```python
from build123d import *

# Parameters (mm, degrees)
SKETCH_1_R          = 2.5
EXTRUDE_1_DEPTH     = 18.5
SKETCH_2_W          = 12
SKETCH_2_H          = 2
EXTRUDE_2_DEPTH     = 18.5
CUT_EXTRUDE_1_REACH = 43.113
SKETCH_3_R          = 2
FILLET_1_R          = 4


with BuildPart() as part:
    # 草图1 → 凸台-拉伸1 (new body)
    with BuildSketch(Plane(origin=(0, 0, 0), x_dir=(1, 0, 0), z_dir=(0, 1, 0))):
        with BuildLine():
            Line((0, -4.5), (16.5, -4.5))
            Line((16.5, -4.5), (16.5, -2.5))
            Line((16.5, -2.5), (3.741657387, -2.5))
            ThreePointArc((3.741657387, -2.5), (-2.121320344, 3.968626967), (0, -4.5))
        make_face()
        with Locations(Location((0, 0, 0), (0, 0, 270))):
            Circle(SKETCH_1_R, mode=Mode.SUBTRACT)
    extrude(amount=EXTRUDE_1_DEPTH)

    # 草图2 → 凸台-拉伸2 (add)
    with BuildSketch(Plane(origin=(0, 18.5, 0), x_dir=(1, 0, 0), z_dir=(0, 1, 0))):
        with Locations((10.5, -3.5)):
            Rectangle(SKETCH_2_W, SKETCH_2_H)
    extrude(amount=EXTRUDE_2_DEPTH)

    # 草图3 → 切除-拉伸1 (cut, up to next)
    with BuildSketch(Plane(origin=(0, 0, 2.5), x_dir=(-1, 0, 0), z_dir=(0, 0, -1)), mode=Mode.PRIVATE) as cut_extrude_1_sk1:
        with Locations((-10.5, 7.5)):
            Circle(SKETCH_3_R)
    cut_extrude_1_tool1 = extrude(cut_extrude_1_sk1.sketch, amount=-CUT_EXTRUDE_1_REACH, mode=Mode.PRIVATE) & part.part
    # 草图3 → 切除-拉伸1 (cut, up to next)
    with BuildSketch(Plane(origin=(0, 0, 2.5), x_dir=(-1, 0, 0), z_dir=(0, 0, -1)), mode=Mode.PRIVATE) as cut_extrude_1_sk2:
        with Locations((-10.5, 29.5)):
            Circle(SKETCH_3_R)
    cut_extrude_1_tool2 = extrude(cut_extrude_1_sk2.sketch, amount=-CUT_EXTRUDE_1_REACH, mode=Mode.PRIVATE) & part.part
    add(cut_extrude_1_tool1.solids().sort_by_distance((10.5, 7.5, 2.5))[0], mode=Mode.SUBTRACT)
    add(cut_extrude_1_tool2.solids().sort_by_distance((10.5, 29.5, 2.5))[0], mode=Mode.SUBTRACT)

    # 圆角1
    fillet_1_edges = [part.edges().sort_by_distance(p)[0] for p in [
        (16.5, 37, 3.5),
        (16.5, 0, 3.5),
    ]]
    fillet(fillet_1_edges, radius=FILLET_1_R)


solid = part.part
```
Can you work these out from the model? Positions are in its coordinate system, mm. A direction names the side the tool comes from. Coordinates: 2 decimals unless noted, no trailing zeros. Loops run counter-clockwise (first coordinate to the right, second up) from the corner with the lowest first, then second, coordinate; pieces in that order, holes last. Notation, with made-up numbers: (14, 74) -> (28, 74) arc R23 ccw to (28, 111) -> close; hole circle Ø10 at (25, 3.5). An arc over 180 degrees is marked (long way). Put each result on its own line as item: value. Start each with the question number.
Q1. I want a section at B-B (y = 29.5). Write out the boundary of the cut face in (x, z), plus the area to 3 significant figures.
Q2. I'm going to push flat-ended pins straight in: P1, Ø3, axis at x = 4.5, z = 0.5, coming from the -Y side; P2, Ø3.5, axis at x = 10.5, y = 29.5, coming from the -Z side; P3, Ø6.5, axis at x = 10.5, y = 7.5, coming from the -Z side; P4, Ø2, axis at y = 29, z = 3.5, coming from the -X side. Where does each tip first touch, or does it pass through?
Q3. For faces 1 (the face through (2, 18.5, 2)), 2 (the face through (15.297, 35.859, 3.486)), which set-ups out of +Z, -Z, +X, -X, +Y, -Y let a thin tool reach every point of the face, with its end or its side?
Q4. I want a section at D-D (z = 3). Write out the boundary of the cut face in (x, y).
Q5. I want a section at A-A (z = 0). Write out the boundary of the cut face in (x, y), plus the area to 3 significant figures.
Q6. If I drill on line 1 (Y direction, x = 10.5, z = 3.7); line 2 (Y direction, x = 9.5, z = 4); line 3 (Z direction, x = 5.5, y = 32), over which ranges is the centre line in solid material (lowest first)? Write a range as [from, to].
Q7. Thinking about a two-plate mould opening in Y: for faces 3 (the face through (10.934, 27.548, 3.486)), 4 (the face through (15.359, 1.203, 3.486)), 5 (the face through (8, 37, 3)), which applies, pulls with the +Y half, pulls with the -Y half, needs draft (parallel to the pull), parting line crosses it, or undercut?
Q8. I want a section at C-C (x = 10.5). Write out the boundary of the cut face in (y, z), plus the area to 3 significant figures.
Taken from the geometry:
1. outline: (4.5, 2.5) -> (8.5, 2.5) -> (8.5, 4.5) -> (4.5, 4.5) -> close; (12.5, 2.5) -> (16.5, 2.5) -> (16.5, 4.5) -> (12.5, 4.5) -> close
1. area: 16.0 mm2
2. P1: stops at y = 0
2. P2: passes through
2. P3: stops at z = 2.5
2. P4: stops at x = 4.5
3. face 1: +Z, -Z, -X, +Y
3. face 2: +Z, -Z, +X, +Y
4. outline: (-3.35, 0) -> (12.5, 0) arc R4 ccw to (16.5, 4) -> (16.5, 33) arc R4 ccw to (12.5, 37) -> (4.5, 37) -> (4.5, 18.5) -> (-3.35, 18.5) -> close; hole circle Ø4 at (10.5, 7.5); hole circle Ø4 at (10.5, 29.5)
5. outline: (-4.5, 0) -> (-2.5, 0) -> (-2.5, 18.5) -> (-4.5, 18.5) -> close; (2.5, 0) -> (4.5, 0) -> (4.5, 18.5) -> (2.5, 18.5) -> close
5. area: 74.0 mm2
6. line 1: y = [0, 5.5], [9.5, 27.5], [31.5, 37]
6. line 2: y = [0, 5.77], [9.23, 27.77], [31.23, 37]
6. line 3: z = [2.5, 4.5]
7. face 3: undercut
7. face 4: pulls with the -Y half
7. face 5: pulls with the +Y half
8. outline: (0, 2.5) -> (5.5, 2.5) -> (5.5, 4.5) -> (0, 4.5) -> close; (9.5, 2.5) -> (27.5, 2.5) -> (27.5, 4.5) -> (9.5, 4.5) -> close; (31.5, 2.5) -> (37, 2.5) -> (37, 4.5) -> (31.5, 4.5) -> close
8. area: 58.0 mm2
